Autodesk Inventor part; units mm, degrees
ref_plane "YZ Plane" through (0, 0, 0) normal (1, 0, 0) x (0, 1, 0)
ref_plane "XZ Plane" through (0, 0, 0) normal (0, 1, 0) x (-1, 0, 0)
ref_plane "XY Plane" through (0, 0, 0) normal (0, 0, 1) x (1, 0, 0)
sketch "Sketch1" plane through (0, 0, 0) normal (0, 1, 0) x (-1, 0, 0)
  line L0 (-160, 60) -> (160, 60)
  line L1 (160, 60) -> (160, -60)
  line L2 (160, -60) -> (-160, -60)
  line L3 (-160, -60) -> (-160, 60)
  line L4 (-160, 60) -> (160, -60) construction
  line L5 (160, 60) -> (-160, -60) construction
  line L6 (-27.6343, -87.1189) -> (-42.3128, -87.1189)
  line L7 (-42.3128, -87.1189) -> (-42.3128, -133.601)
  line L8 (-42.3128, -133.601) -> (-27.6343, -133.601)
  line L9 (-27.6343, -133.601) -> (-27.6343, -87.1189)
  line L10 (-27.6343, -87.1189) -> (-42.3128, -133.601) construction
  line L11 (-42.3128, -87.1189) -> (-27.6343, -133.601) construction
  point P0 (0, 0)
  point P1 (-34.9736, -110.3599)
  dimension "d0" = 320
  dimension "d1" = 120
extrude "Extrusion1" add sketch "Sketch1" along normal blind 10 contours L0 L1 L2 L3
sketch "Sketch2" plane through (0, 10, 0) normal (0, 1, 0) x (1, 0, 0)
  line L0 (-160, -60) -> (160, -60)
  line L1 (-160, -60) -> (66.1592, -60)
  line L2 (66.1592, -60) -> (66.1592, -55.6043)
  line L3 (66.1592, -55.6043) -> (-160, -55.6043)
  line L4 (-160, -55.6043) -> (-160, -60)
  point P0 (0, 0)
extrude "Extrusion2" add sketch "Sketch2" along normal blind 50
sketch "Sketch3" plane through (0, 10, 0) normal (0, 1, 0) x (1, 0, 0)
  line L0 (-160, 60) -> (-160, -60)
  line L1 (-160, 60) -> (68.4346, 60)
  line L2 (68.4346, 60) -> (68.4346, 56.0614)
  line L3 (68.4346, 56.0614) -> (-160, 56.0614)
  line L4 (-160, 56.0614) -> (-160, 60)
  point P0 (0, 0)
extrude "Extrusion3" add sketch "Sketch3" along normal blind 50
sketch "Sketch4" plane through (-160, 0, -60) normal (-1, 0, 0) x (0, 0, 1)
  line L0 (120, -68.4573) -> (0, -68.4573)
  line L1 (0, -68.4573) -> (0, 81.272)
  line L2 (0, 81.272) -> (120, 81.272)
  line L3 (120, 81.272) -> (120, -68.4573)
  line L4 (120, -68.4573) -> (0, 81.272) construction
  line L5 (0, -68.4573) -> (120, 81.272) construction
  point P0 (60, 0)
  point P1 (60, 6.4073)
extrude "Extrusion4" add sketch "Sketch4" along normal blind 5
sketch "Sketch5" plane through (-165, 0, -60) normal (-1, 0, 0) x (0, 0, 1)
  line L0 (120, -68.4573) -> (120, 81.272)
  line L1 (0, 0) -> (120, 0)
  line L2 (120, 0) -> (120, -68.4573)
  line L3 (120, -68.4573) -> (0, -68.4573)
  line L4 (0, -68.4573) -> (0, 0)
  point P0 (60, 0)
extrude "Extrusion5" cut sketch "Sketch5" against normal blind 5
sketch "Sketch6" plane through (160, 0, -60) normal (0, 0, -1) x (-1, 0, 0)
  line L0 (91.5654, 10) -> (91.5654, 60)
  line L1 (0, 0) -> (0, 10)
  line L2 (91.5654, 60) -> (0, 60)
  line L3 (0, 60) -> (0, 10)
  line L4 (0, 10) -> (91.5654, 10)
  line L5 (91.5654, 10) -> (91.5654, 60)
  point P0 (160, 0)
extrude "Extrusion6" add sketch "Sketch6" against normal blind 5
sketch "Sketch7" plane through (160, 0, 60) normal (0, 0, 1) x (1, 0, 0)
  line L0 (-93.8408, 10) -> (-93.8408, 60)
  line L1 (0, 0) -> (0, 60)
  line L2 (-93.8408, 60) -> (0, 60)
  line L3 (0, 60) -> (0, 9.1052)
  line L4 (0, 9.1052) -> (-93.8408, 9.1052)
  line L5 (-93.8408, 9.1052) -> (-93.8408, 60)
  point P0 (-160, 0)
extrude "Extrusion7" cut sketch "Sketch7" against normal blind 5
sketch "Sketch8" plane through (-160, 60, 60) normal (0, 0, 1) x (1, 0, 0)
  line L0 (320, -50) -> (228.4346, -50)
  line L1 (226.1592, 0) -> (320, 0)
  line L2 (320, 0) -> (320, -50)
  line L3 (320, -50) -> (226.1592, -50)
  line L4 (226.1592, -50) -> (226.1592, 0)
  point P0 (160, -60)
extrude "Extrusion8" add sketch "Sketch8" against normal blind 5
sketch "Sketch9" plane through (160, 0, -60) normal (0, 0, -1) x (-1, 0, 0)
  line L0 (93.8408, 10) -> (93.8408, 60)
  line L1 (0, 10) -> (91.5654, 10)
  line L2 (93.8408, 60) -> (0, 10)
  line L3 (0, 10) -> (0, 60)
  line L4 (0, 60) -> (93.8408, 60)
  point P0 (160, 0)
extrude "Extrusion9" cut sketch "Sketch9" against normal blind 5
sketch "Sketch10" plane through (-160, 60, 55) normal (0, 0, -1) x (-1, 0, 0)
  point P0 (-160, -60)
sketch "Sketch11" plane through (-160, 60, 60) normal (0, 0, 1) x (1, 0, 0)
  line L0 (228.4346, -50) -> (228.4346, 0)
  line L1 (0, 0) -> (320, 0)
  line L2 (320, -50) -> (320, 0)
  line L3 (320, -50) -> (228.4346, -1.2124)
  line L4 (320, -50) -> (228.4346, -1.2124)
  line L5 (228.4346, -1.2124) -> (228.4346, -50)
  line L6 (320, -60) -> (-5, -60)
  point P0 (160, -60)
extrude "Extrusion10" cut sketch "Sketch11" against normal blind 5
properties part number "Storagecontainer"
Check sheet for the modelled part. Datum: model origin and axes. Units: mm. A direction names the side the tool comes from. Round coordinates to 2 decimals unless told otherwise and drop trailing zeros. Loops run counter-clockwise (first coordinate to the right, second up) from the corner with the lowest first, then second, coordinate; pieces in that order, holes last. Notation, with made-up numbers: M 9.5,6 L 46.5,6 A12 ccw 46.5,14 Z; hole C -38.5,-5.5 d9. An arc over 180 degrees is marked long. Answer as a JSON object with one key per item and string values.
1. Access from +Z, -Z, +X, -X, +Y, -Y to the whole of each face (thin tool, end or side, straight path). Record for faces 1 (the flat face through (95, 24, -55)), 2 (the flat face through (-165, 41, -1)), 3 (the flat face through (-45, 35, 55.604)).
Reply:
{"face 1": "+X, +Y", "face 2": "+Z, -Z, -X, +Y, -Y", "face 3": "+Y"}
2. Section check D-D (z = -14.5). Record the boundary of the cut face in (x, y), plus the area to 3 significant figures.
Reply:
{"outline": "M -165,0 L 160,0 L 160,10 L -160,10 L -160,81.27 L -165,81.27 Z", "area": "3,610 mm²"}
3. Section check B-B (x = -94). Record the boundary of the cut face in (y, z), plus the area to 3 significant figures.
Reply:
{"outline": "M 0,-60 L 60,-60 L 60,-56.06 L 10,-56.06 L 10,55.6 L 60,55.6 L 60,60 L 0,60 Z", "area": "1,620 mm²"}
4. Scan lines: line 1 (Z direction, x = 104.5, y = 15.5); line 2 (Z direction, x = 50.5, y = 58); line 3 (X direction, y = 28.5, z = -41). Record each from-to range of solid material in increasing order.
Reply:
{"line 1": "z = -60 to -55, 55 to 60", "line 2": "z = -60 to -56.06, 55.6 to 60", "line 3": "x = -165 to -160"}
5. Mould release check, pull along Z, two halves, no side actions. Record for faces 4 (the flat face through (-36, 32, -60)), 5 (the flat face through (92, 24, 55)), 6 (the flat face through (0, 0, 1)): pulls with the +Z half, pulls with the -Z half, needs draft (parallel to the pull), parting line crosses it, or undercut.
Reply:
{"face 4": "pulls with the -Z half", "face 5": "undercut", "face 6": "needs draft"}
6. Gauge pin test, flat ends, axial feed: P1, Ø1, axis at y = 59, z = 57.5, coming from the +X side; P2, Ø3, axis at x = -14, z = -58, coming from the +Y side; P3, Ø10, axis at y = 62, z = -30.5, coming from the +X side. Record the tip position at first contact, or that the pin passes through.
Reply:
{"P1": "stops at x = 68.97", "P2": "stops at y = 60", "P3": "stops at x = -160"}
7. Section check C-C (y = 40). Record the boundary of the cut face in (x, z).
Reply:
{"outline": "M -165,-60 L 103.7,-60 L 103.7,-55 L 68.43,-55 L 68.43,-56.06 L -160,-56.06 L -160,55.6 L 66.16,55.6 L 66.16,55 L 103.7,55 L 103.7,60 L -165,60 Z"}
